```python
from build123d import *

# Parameters (mm, degrees)
F0_R     = 65
F1_DEPTH = 20
F2_T     = -5
F3_R     = 2.5


with BuildPart() as f1:
    # F0 (on Top) → F1 (new body)
    with BuildSketch(Plane.XY):
        Circle(F0_R)
    extrude(amount=F1_DEPTH)

    # F2
    f2_openings = [f1.faces().sort_by_distance(p)[0] for p in [
        (0, 0, 0),
    ]]
    offset(amount=F2_T, openings=f2_openings)

    # F3
    f3_edges = [f1.edges().sort_by_distance(p)[0] for p in [
        (-65, 0, 20),
    ]]
    fillet(f3_edges, radius=F3_R)


solid = f1.part
```
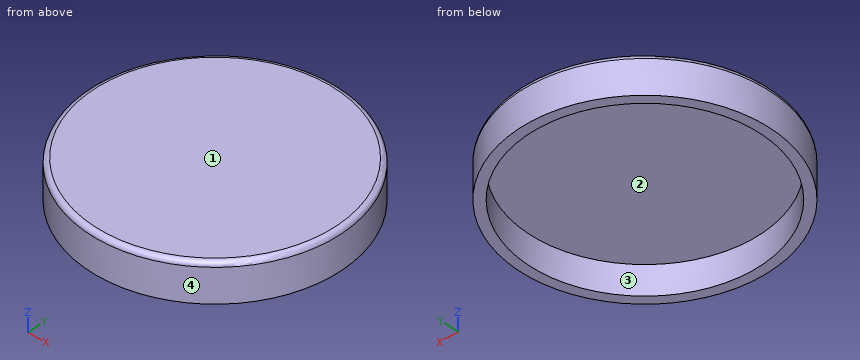
CAD build for the part. Positions are in the model's coordinates, mm. Face numbers are marked on the shaded views. Coordinates: 2 decimals unless noted, no trailing zeros. Order: outer loops, then holes, each group sorted by start corner. A loop starts at its lowest first (then second) coordinate and runs counter-clockwise, first axis right, second up. Notation, with made-up numbers: (42.5, -18) - (93.5, -18) arc R31 cw to (93.5, 14) - close; hole circle Ø3 at (19.5, 58.25). An arc over 180 degrees is marked (long way). Answer in a Markdown table with one row per item.
1. Pull direction X, two halves, no side cores. Call the marked faces 1, 2, 3 and 4: +X half, -X half, draft (parallel to the pull), parting line (faces both ways), or undercut.
Answer:
| item | result |
|---|---|
| face 1 | draft |
| face 2 | undercut |
| face 3 | undercut |
| face 4 | parting line |
2. Drill centre lines: L1, parallel to Y at x = 0, z = 5.5; L2, parallel to Z at x = 32, y = 41; L3, parallel to Y at x = -13.5, z = 13. Where is each one in solid material? Low to high. Write a range as from..to.
Answer:
| item | result |
|---|---|
| L1 | -65..-60, 60..65 |
| L2 | 15..20 |
| L3 | -63.58..-58.46, 58.46..63.58 |
3. Slice it at C-C, the plane z = 8. List the corners of the cut face in (x, y).
Answer:
| item | result |
|---|---|
| outline | circle Ø130 at (0, 0); hole circle Ø120 at (0, 0) |
4. Slice it at A-A, the plane x = 0. List the corners of the cut face in (y, z).
Answer:
| item | result |
|---|---|
| outline | (-65, 0) - (-60, 0) - (-60, 15) - (60, 15) - (60, 0) - (65, 0) - (65, 17.5) arc R2.5 ccw to (62.5, 20) - (-62.5, 20) arc R2.5 ccw to (-65, 17.5) - close |
5. Flat gauge pins, fed straight in: P1, Ø8, axis at x = 44, y = 11, coming from the -Z side; P2, Ø5, axis at x = 51.5, z = 15, coming from the -Y side; P3, Ø6, axis at y = 11.5, z = 3.5, coming from the -X side. Where does each tip first touch, or does it go through?
Answer:
| item | result |
|---|---|
| P1 | z = 15 |
| P2 | y = -42.71 |
| P3 | x = -64.44 |
